```python
from build123d import *

# Parameters (mm, degrees)
RESSALTO_EXTRUS_O1_DEPTH = 10
ESBO_O6_R                = 4
CORTE_EXTRUS_O2_DEPTH    = 30.478805946


with BuildPart() as part:
    # Esboço2 → Ressalto-extrusão1 (new body)
    with BuildSketch(Plane(origin=(0, 0, 0), x_dir=(0, 0, -1), z_dir=(1, 0, 0))):
        Polygon((0, 0), (25, 0), (25, 7), (20, 7), (20, 12), (5, 12), (5, 7), (0, 7), align=None)
    extrude(amount=RESSALTO_EXTRUS_O1_DEPTH)

    # Esboço6 → Corte-extrusão2 (cut, through all)
    with BuildSketch(Plane(origin=(0, 12, 0), x_dir=(1, 0, 0), z_dir=(0, 1, 0))):
        with Locations(Location((5, 12.5, 0), (0, 0, 270))):
            Circle(ESBO_O6_R)
    extrude(amount=-CORTE_EXTRUS_O2_DEPTH, mode=Mode.SUBTRACT)


solid = part.part
```
Input: part model. Units: mm. Frame: model coordinates. A direction names the side the tool comes from. Round coordinates to 2 decimals unless told otherwise and drop trailing zeros. Loops run counter-clockwise (first coordinate to the right, second up) from the corner with the lowest first, then second, coordinate; pieces in that order, holes last. Notation, with made-up numbers: (-39.75, -39) -> (-4.75, -39) arc R24 ccw to (-4.75, -21) -> close; hole circle Ø9 at (81.5, 53.5). An arc over 180 degrees is marked (long way). Use one line per item in the form item = value. Start each with the question number.
Item 1: Section query A-A on x = 5. Return the cut outline in (y, z).
Item 2: Section query D-D on x = 3.75. Return the cut outline in (y, z), then the cut area to 3 significant figures.
Item 3: Section query C-C on y = 10.5. Return the cut outline in (x, z).
Item 4: Contact query for flat-ended pins moving along their axis: pin 1 Ø2 at (x, y) = (8.5, 9.5) entering from +Z; pin 2 Ø2.5 at (x, z) = (3.5, -2) entering from +Y; pin 3 Ø2.5 at (x, y) = (7.5, 9) entering from -Z. Output: stop coordinate, or through.
Item 5: Section query B-B on z = -12.5. Return the cut outline in (x, y).
Item 6: Material intervals for L1, parallel to X at y = 2.75, z = -12.5; L2, parallel to Y at x = 1.25, z = -21.75; L3, parallel to X at y = 3, z = -14.25, sorted ascending. Write a range as from..to.
Item 7: Set-up query: faces 5 (the face through (0, 5, -12)), 6 (the face through (5, 9, -20)), 7 (the face through (5, 10, -5)). Return all of +Z, -Z, +X, -X, +Y, -Y with unobstructed straight access to the full face (end or side cutting, diameter ignored); none if empty.
Item 8: Mould query, pull axis Z, two halves, no side actions, for faces 1 (the face through (5, 7, -23)), 2 (the face through (5, 3, -25)), 3 (the face through (2.6, 6.1, -15.7)), 4 (the face through (5, 4, 0)). Classes: pulls with the +Z half, pulls with the -Z half, needs draft (parallel to the pull), parting line crosses it, or undercut.
Ans:
q1.outline = (0, -25) -> (7, -25) -> (7, -20) -> (12, -20) -> (12, -16.5) -> (0, -16.5) -> close; (0, -8.5) -> (12, -8.5) -> (12, -5) -> (7, -5) -> (7, 0) -> (0, 0) -> close
q2.outline = (0, -25) -> (7, -25) -> (7, -20) -> (12, -20) -> (12, -16.3) -> (0, -16.3) -> close; (0, -8.7) -> (12, -8.7) -> (12, -5) -> (7, -5) -> (7, 0) -> (0, 0) -> close
q2.area = 159 mm^2
q3.outline = (0, -20) -> (10, -20) -> (10, -5) -> (0, -5) -> close; hole circle Ø8 at (5, -12.5)
q4.pin_1 = -5
q4.pin_2 = 7
q4.pin_3 = -20
q5.outline = (0, 0) -> (1, 0) -> (1, 12) -> (0, 12) -> close; (9, 0) -> (10, 0) -> (10, 12) -> (9, 12) -> close
q6.L1 = 0..1, 9..10
q6.L2 = 0..7
q6.L3 = 0..1.4, 8.6..10
q7.face_5 = +Z, -Z, -X, +Y, -Y
q7.face_6 = -Z, +X, -X, +Y
q7.face_7 = +Z, +X, -X, +Y
q8.face_1 = needs draft
q8.face_2 = pulls with the -Z half
q8.face_3 = undercut
q8.face_4 = pulls with the +Z half
